Could you check a few things on this model? Use its own coordinates, in mm. Give positions to 0.01 mm unless a question says otherwise; leave off trailing zeros. Loops run counter-clockwise (first coordinate to the right, second up) from the corner with the lowest first, then second, coordinate; pieces in that order, holes last. Notation, with made-up numbers: (89, 52) -> (136, 52) arc R24 ccw to (136, 70) -> close; hole circle Ø7 at (14, -31). An arc over 180 degrees is marked (long way). Write item = value, one per line. Start each with the question number.
1) I want a section at C-C (z = -31). List the corners of the cut face in (x, y) for me, and give its area (3 significant figures).
2) I want a section at B-B (y = 1.3). List the corners of the cut face in (x, z) for me.
3) I want a section at A-A (x = -107.5). List the corners of the cut face in (y, z) for me, and give its area (3 significant figures).
4) I'm going to push flat-ended pins straight in: pin 1 Ø2 at (x, z) = (-86, -8.5) entering from +Y; pin 2 Ø0.6 at (x, y) = (-77, 0.5) entering from +Z; pin 3 Ø1 at (x, y) = (-58.5, 1) entering from -Z. Where does each tip first touch, or does it pass through?
5) I need wall thicknesses on probe 1 along Z at (x, y) = (-35, 0.9); probe 2 along X at (y, z) = (1.9, -93); probe 3 along X at (y, z) = (1.1, 16). Which ranges of each line are inside material? Lowest first, please. Write a range as from..to.
from build123d import *

# Parameters (mm, degrees)
SKETCH_1_R          = 1.6
EXTRUDE_1_DEPTH     = 2
EXTRUDE_2_DEPTH     = 2
CUT_EXTRUDE_1_DEPTH = 193.473374782
FILLET_1_R          = 2


with BuildPart() as part:
    # 草图1 → 凸台-拉伸1 (new body)
    with BuildSketch(Plane(origin=(0, 0, 0), x_dir=(1, 0, 0), z_dir=(0, 1, 0))):
        with BuildLine():
            Line((-28, -16), (-28, 0))
            Line((-28, 0), (-131, 0))
            Line((-131, 0), (-131, 133))
            Line((-131, 133), (0, 133))
            Line((0, 133), (0, 0))
            Line((0, 0), (-8.852716607, -20.040693817))
            ThreePointArc((-8.852716607, -20.040693817), (-20.064844554, -25.78449881), (-28, -16))
        make_face()
        with Locations(Location((-18, -9, 0), (0, 0, 270))):
            Circle(SKETCH_1_R, mode=Mode.SUBTRACT)
        with Locations(Location((-11, -16, 0), (0, 0, 270))):
            Circle(SKETCH_1_R, mode=Mode.SUBTRACT)
        with Locations(Location((-18, -23, 0), (0, 0, 270))):
            Circle(SKETCH_1_R, mode=Mode.SUBTRACT)
        with Locations(Location((-25, -16, 0), (0, 0, 270))):
            Circle(SKETCH_1_R, mode=Mode.SUBTRACT)
        with Locations(Location((-18, -16, 0), (0, 0, 270))):
            Circle(SKETCH_1_R, mode=Mode.SUBTRACT)
    extrude(amount=EXTRUDE_1_DEPTH)

    # 草图2 → 凸台-拉伸2 (add)
    with BuildSketch(Plane(origin=(0, 2, 0), x_dir=(1, 0, 0), z_dir=(0, 1, 0))):
        Polygon((-131, 133), (-131, 141), (-121, 141), (-126, 137), (-126, 135), (-121, 133), align=None)
    extrude(amount=-EXTRUDE_2_DEPTH)

    # 草图3 → 切除-拉伸1 (cut, through all)
    with BuildSketch(Plane(origin=(0, 2, 0), x_dir=(1, 0, 0), z_dir=(0, 1, 0))):
        with BuildLine():
            Line((-124, 128), (-9, 128))
            ThreePointArc((-9, 128), (-7.585786438, 127.414213562), (-7, 126))
            Line((-7, 126), (-7, 9))
            ThreePointArc((-7, 9), (-7.585786438, 7.585786438), (-9, 7))
            Line((-9, 7), (-124, 7))
            ThreePointArc((-124, 7), (-125.414213562, 7.585786438), (-126, 9))
            Line((-126, 9), (-126, 126))
            ThreePointArc((-126, 126), (-125.414213562, 127.414213562), (-124, 128))
        make_face()
    extrude(amount=-CUT_EXTRUDE_1_DEPTH, mode=Mode.SUBTRACT)

    # 圆角1
    fillet_1_edges = [part.edges().sort_by_distance(p)[0] for p in [
        (-28, 1, 0),
        (-131, 1, 0),
        (0, 1, -133),
    ]]
    fillet(fillet_1_edges, radius=FILLET_1_R)


solid = part.part
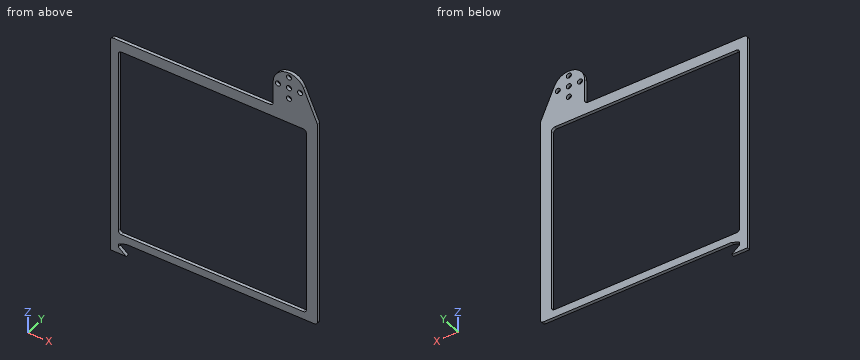
Answer list:
q1.outline = (-131, 0) -> (-126, 0) -> (-126, 2) -> (-131, 2) -> close; (-7, 0) -> (0, 0) -> (0, 2) -> (-7, 2) -> close
q1.area = 24.0 mm^2
q2.outline = (-131, -141) -> (-121, -141) -> (-126, -137) -> (-126, -135) -> (-121, -133) -> (-2, -133) arc R2 ccw to (0, -131) -> (0, 0) -> (-8.85, 20.04) arc R10 ccw to (-28, 16) -> (-28, 2) arc R2 cw to (-30, 0) -> (-129, 0) arc R2 ccw to (-131, -2) -> close; hole (-126, -126) arc R2 ccw to (-124, -128) -> (-9, -128) arc R2 ccw to (-7, -126) -> (-7, -9) arc R2 ccw to (-9, -7) -> (-124, -7) arc R2 ccw to (-126, -9) -> close; hole circle Ø3.2 at (-25, 16); hole circle Ø3.2 at (-18, 9); hole circle Ø3.2 at (-18, 16); hole circle Ø3.2 at (-18, 23); hole circle Ø3.2 at (-11, 16)
q3.outline = (0, -133) -> (2, -133) -> (2, -128) -> (0, -128) -> close; (0, -7) -> (2, -7) -> (2, 0) -> (0, 0) -> close
q3.area = 24.0 mm^2
q4.pin_1 = through
q4.pin_2 = 0
q4.pin_3 = -133
q5.probe_1 = -133..-128, -7..0
q5.probe_2 = -131..-126, -7..0
q5.probe_3 = -28..-26.6, -23.4..-19.6, -16.4..-12.6, -9.4..-7.07
